CAD build for the part. Positions are in the model's coordinates, mm. Face numbers are marked on the shaded views. A direction names the side the tool comes from. Round coordinates to 2 decimals unless told otherwise and drop trailing zeros. Order: outer loops, then holes, each group sorted by start corner. A loop starts at its lowest first (then second) coordinate and runs counter-clockwise, first axis right, second up.
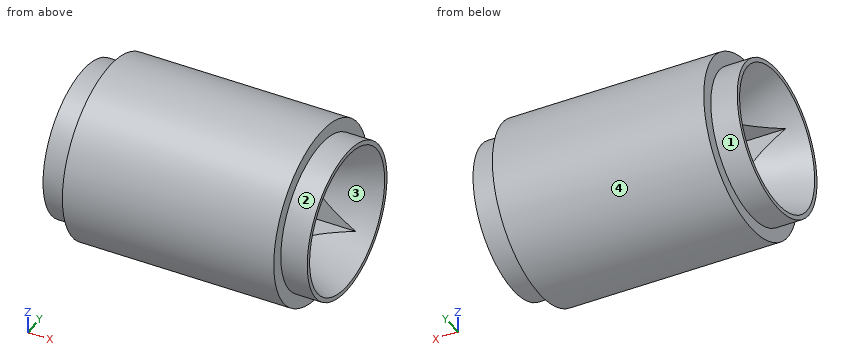
Autodesk Inventor part; units mm, degrees
ref_plane "YZ Plane" through (0, 0, 0) normal (1, 0, 0) x (0, 1, 0)
ref_plane "XZ Plane" through (0, 0, 0) normal (0, 1, 0) x (-1, 0, 0)
sketch "Szkic1" plane through (0, 0, 0) normal (0, 0, 1) x (1, 0, 0)
  point P0 (0, 0)
sketch "Szkic2" plane through (0, 0, 0) normal (0, 0, 1) x (1, 0, 0)
  line L0 (-26.25, 0) -> (-26.25, 8.5)
  line L1 (-26.25, 8.5) -> (-23.25, 8.5)
  line L2 (-23.25, 8.5) -> (-23.25, 10)
  line L3 (-23.25, 10) -> (0.75, 10)
  line L4 (0.75, 10) -> (0.75, 8.5)
  line L5 (0.75, 8.5) -> (3.75, 8.5)
  line L6 (3.75, 8.5) -> (3.75, 0)
  line L7 (3.75, 0) -> (-26.25, 0)
  point P0 (0, 0)
  dimension "d0" = 30
  dimension "d2" = 3
  dimension "d3" = 24
  dimension "d4" = 20
  dimension "d5" = 17
revolve "Obrót1" add sketch "Szkic2" angle 360 about axis through (3.75, 0, 0) along (-1, 0, 0)
sketch "Szkic3" plane through (3.75, 0, 0) normal (1, 0, 0) x (0, 0, -1)
  circle A0 centre (0, 0) radius 8
  dimension "d7" = 16
extrude "Wyciągnięcie proste1" cut sketch "Szkic3" against normal blind 10 draft -24
sketch "Szkic4" plane through (-26.25, 0, 0) normal (-1, 0, 0) x (0, 0, 1)
  line L0 (-5.1, -5.1) -> (5.1, -5.1)
  line L1 (5.1, -5.1) -> (5.1, 5.1)
  line L2 (5.1, 5.1) -> (-5.1, 5.1)
  line L3 (-5.1, 5.1) -> (-5.1, -5.1)
  line L4 (-5.1, -5.1) -> (5.1, 5.1) construction
  line L5 (5.1, -5.1) -> (-5.1, 5.1) construction
  point P0 (0, 0)
  dimension "d10" = 10.2
  dimension "d11" = 10.2
extrude "Wyciągnięcie proste2" cut sketch "Szkic4" against normal through all
sketch "Szkic5" plane through (-26.25, 0, 0) normal (-1, 0, 0) x (0, 0, 1)
  circle A0 centre (0, 0) radius 8
  dimension "d14" = 16
extrude "Wyciągnięcie proste3" cut sketch "Szkic5" against normal blind 10 draft -24
sketch "Szkic6" plane through (0, 0, 0) normal (0, 0, 1) x (1, 0, 0)
  point P0 (0, 0)
properties part number "Bartosz_Zukowski_model_nr_13"
1. Mould opens along Y. For the marked faces 3 and 4 say: released by +Y, released by -Y, zero draft, split by the parting line, or undercut.
2. Pin check, flat tips, straight feed: P1, Ø1, axis at x = -2.5, z = 4.5, coming from the -Y side; P2, Ø5, axis at x = -5.5, z = 5.5, coming from the -Y side; P3, Ø1.5, axis at x = -11.5, z = -5, coming from the -Y side. Stop position of each tip, or through.
3. Cut at D-D, the plane x = -2. Write the cut outline in (y, z), and give its area (3 significant figures).
4. Tool access for the marked faces 1 and 2: list every direction of +Z, -Z, +X, -X, +Y, -Y with a clear straight run to the whole face (end or side of a thin tool).
5. Cut at A-A, the plane y = 0. Write the cut outline in (x, z).
6. Cut at B-B, the plane x = -18.75. Write the cut outline in (y, z), and give its area (3 significant figures).
7. Drill centre lines: line 1 (Z direction, x = -12.75, y = -6); line 2 (Y direction, x = -5.5, z = 5); line 3 (Z direction, x = -11.25, y = -1.5). Where is each one in solid material? Low to high.
Outcome:
1. face 3: undercut
1. face 4: split by the parting line
2. P1: stops at y = -9.17
2. P2: stops at y = -9.54
2. P3: stops at y = -9.05
3. outline: circle Ø20 at (0, 0); hole (-5.1, -5.1) - (-1.89, -5.1) arc R5.44 ccw to (1.89, -5.1) - (5.1, -5.1) - (5.1, -1.89) arc R5.44 ccw to (5.1, 1.89) - (5.1, 5.1) - (1.89, 5.1) arc R5.44 ccw to (-1.89, 5.1) - (-5.1, 5.1) - (-5.1, 1.89) arc R5.44 ccw to (-5.1, -1.89) - close
3. area: 207 mm2
4. face 1: -X
4. face 2: +X
5. outline: (-26.25, -8.5) - (-23.25, -8.5) - (-23.25, -10) - (0.75, -10) - (0.75, -8.5) - (3.75, -8.5) - (3.75, -8) - (-2.76, -5.1) - (-19.74, -5.1) - (-26.25, -8) - close; (-26.25, 8) - (-19.74, 5.1) - (-2.76, 5.1) - (3.75, 8) - (3.75, 8.5) - (0.75, 8.5) - (0.75, 10) - (-23.25, 10) - (-23.25, 8.5) - (-26.25, 8.5) - close
6. outline: circle Ø20 at (0, 0); hole (-5.1, -5.1) - (5.1, -5.1) - (5.1, 5.1) - (-5.1, 5.1) - close
6. area: 210 mm2
7. line 1: z = -8 to 8
7. line 2: y = -8.66 to -5.1, 5.1 to 8.66
7. line 3: z = -9.89 to -5.1, 5.1 to 9.89
